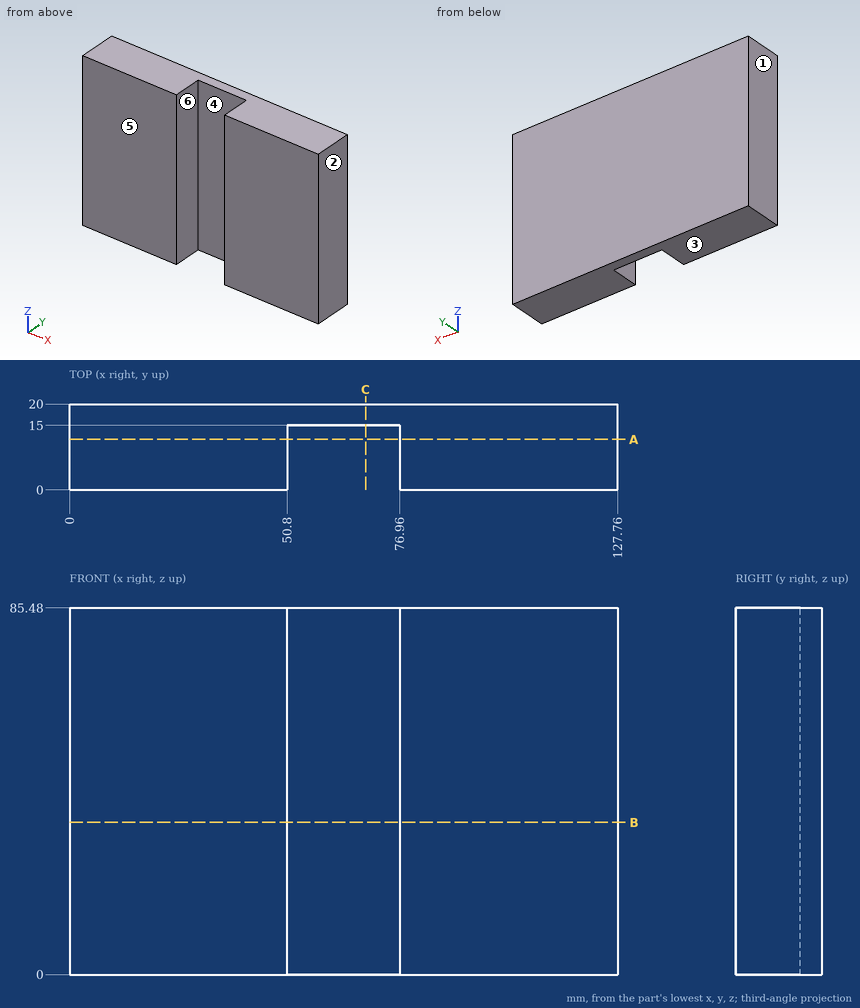
Drawing for the job (mm, zero at the part's lowest x, y, z). A direction names the side the tool comes from. Round coordinates to 2 decimals unless told otherwise and drop trailing zeros. Write each loop counter-clockwise with the first axis right and the second up, starting at its lowest first coordinate (ties: lowest second). Pieces come first, ordered by that corner, then holes. Notation, with made-up numbers: (38, 8) - (79, 8) arc R24 cw to (79, 36) - close; hole circle Ø6 at (77.25, 50.5). An arc over 180 degrees is marked (long way). Use CSV: the item, a comma, the result in double quotes.
(1) Band-saw the part on B-B (z = 35.5). Write the cut outline in (x, y), plus the area to 3 significant figures.
Response:
outline,"(0, 0) - (50.8, 0) - (50.8, 15) - (76.96, 15) - (76.96, 0) - (127.76, 0) - (127.76, 20) - (0, 20) - close"
area,"2,160 mm²"
(2) 3-axis set-ups, long thin cutter, end or side, ignore diameter. For the marked faces 5 and 6: which of +Z, -Z, +X, -X, +Y, -Y reach the whole face in a straight line?
Response:
face 5,"+Z, -Z, +X, -X, -Y"
face 6,"+Z, -Z, -Y"
(3) Band-saw the part on A-A (y = 11.75). Write the cut outline in (x, z), plus the area to 3 significant figures.
Response:
outline,"(0, 0) - (50.8, 0) - (50.8, 85.48) - (0, 85.48) - close; (76.96, 0) - (127.76, 0) - (127.76, 85.48) - (76.96, 85.48) - close"
area,"8,680 mm²"
(4) Pin check, flat tips, straight feed: P1, Ø5, axis at x = 63.5, z = 35.5, coming from the -Y side; P2, Ø6, axis at x = 56, y = 7.5, coming from the +Z side. Stop position of each tip, or through.
Response:
P1,"y = 15"
P2,"through"
(5) Mould opens along X. For the marked faces 1, 2, 3 and 4 say: pulls with the +X half, pulls with the -X half, needs draft (parallel to the pull), parting line crosses it, or undercut.
Response:
face 1,"pulls with the -X half"
face 2,"pulls with the +X half"
face 3,"needs draft"
face 4,"undercut"
(6) Wall check: line 1 (X direction, y = 6.5, z = 26.5); line 2 (Y direction, x = 62.5, z = 36). Give the ranges that are in metal, low to high.
Response:
line 1,"0 to 50.8, 76.96 to 127.76"
line 2,"15 to 20"
(7) Band-saw the part on C-C (x = 69). Write the cut outline in (y, z), plus the area to 3 significant figures.
Response:
outline,"(15, 0) - (20, 0) - (20, 85.48) - (15, 85.48) - close"
area,"427 mm²"
